Design review of the part built by this model. Coordinates are the model's own, in mm. A direction names the side the tool comes from. Coordinates: 2 decimals unless noted, no trailing zeros. Order: outer loops, then holes, each group sorted by start corner. A loop starts at its lowest first (then second) coordinate and runs counter-clockwise, first axis right, second up. Notation, with made-up numbers: M 31,63 L 58,63 A25 cw 58,78 Z; hole C 23,-19 d5. An arc over 180 degrees is marked long. Answer in a Markdown table with one row per item.
from build123d import *

# Parameters (mm, degrees)
F0_W          = 6
F0_H          = 1.5
F1_DEPTH      = 22
F2_R          = 2.5
F3_DEPTH      = 25
F3_DEPTH_BACK = 25
F4_START      = 0.5
F2_R_2        = 5
F2_R_3        = 4
F4_DEPTH      = 24.5
F2_R_4        = 1.5
F5_DEPTH      = 25
F5_DEPTH_BACK = 25
F6_DEPTH      = 25
F6_DEPTH_BACK = 1.5
F7_START      = -4
F7_DEPTH      = 21


with BuildPart() as f1:
    # F0 (on Front) → F1 (new body)
    with BuildSketch(Plane.XZ):
        with Locations((0, -4.75)):
            Rectangle(F0_W, F0_H)
        Polygon((3, -4), (10, -4), (10, 4), (-10, 4), (-10, -4), (-3, -4), align=None)
    extrude(amount=F1_DEPTH)

    # F2 (on Top) → F3 (cut, two sides)
    with BuildSketch(Plane.XY) as f3_sk:
        with Locations((0, -6.5)):
            Circle(F2_R)
    extrude(amount=F3_DEPTH, mode=Mode.SUBTRACT)
    extrude(f3_sk.sketch, amount=-F3_DEPTH_BACK, mode=Mode.SUBTRACT)

    # F2 (on Top) → F4 (cut)
    with BuildSketch(Plane.XY.offset(F4_START)):
        with Locations((0, -6.5)):
            Circle(F2_R_2)
        with Locations((0, -6.5)):
            Circle(F2_R_3, mode=Mode.SUBTRACT)
        with Locations((0, -6.5)):
            Circle(F2_R_3)
        with Locations((0, -6.5)):
            Circle(F2_R, mode=Mode.SUBTRACT)
    extrude(amount=F4_DEPTH, mode=Mode.SUBTRACT)

    # F2 (on Top) → F5 (cut, two sides)
    with BuildSketch(Plane.XY) as f5_sk:
        with Locations((-4.685, -17.2488261014)):
            Circle(F2_R_4)
        with Locations((4.685, -17.2488261014)):
            Circle(F2_R_4)
    extrude(amount=F5_DEPTH, mode=Mode.SUBTRACT)
    extrude(f5_sk.sketch, amount=-F5_DEPTH_BACK, mode=Mode.SUBTRACT)

    # F2 (on Top) → F6 (cut, two sides)
    with BuildSketch(Plane.XY) as f6_sk:
        Polygon((-1.85, -18.8856141146), (-1.85, -15.6120380883), (-4.685, -13.9752500751), (-7.52, -15.6120380883), (-7.52, -18.8856141146), (-4.685, -20.5224021277), align=None)
        with Locations((-4.685, -17.2488261014)):
            Circle(F2_R_4, mode=Mode.SUBTRACT)
        Polygon((7.52, -18.8856141146), (7.52, -15.6120380883), (4.685, -13.9752500751), (1.85, -15.6120380883), (1.85, -18.8856141146), (4.685, -20.5224021277), align=None)
        with Locations((4.685, -17.2488261014)):
            Circle(F2_R_4, mode=Mode.SUBTRACT)
    extrude(amount=-F6_DEPTH, mode=Mode.SUBTRACT)
    extrude(f6_sk.sketch, amount=F6_DEPTH_BACK, mode=Mode.SUBTRACT)

    # F2 (on Top) → F7 (cut)
    with BuildSketch(Plane.XY.offset(F7_START)):
        with Locations((0, -6.5)):
            Circle(F2_R_3)
        with Locations((0, -6.5)):
            Circle(F2_R, mode=Mode.SUBTRACT)
    extrude(amount=-F7_DEPTH, mode=Mode.SUBTRACT)


solid = f1.part
(1) Add section B-B, the plane z = -2. Give the boundary of the cut face in (x, y) (3 decimals).
Return value:
| item | result |
|---|---|
| outline | M -10,-22 L 10,-22 L 10,0 L -10,0 Z; hole M -7.52,-18.886 L -4.685,-20.522 L -1.85,-18.886 L -1.85,-15.612 L -4.685,-13.975 L -7.52,-15.612 Z; hole C 0,-6.5 d5; hole M 1.85,-18.886 L 4.685,-20.522 L 7.52,-18.886 L 7.52,-15.612 L 4.685,-13.975 L 1.85,-15.612 Z |
(2) Add section C-C, the plane y = -6.5. Give the boundary of the cut face in (x, z), and give its area (4 significant figures).
Return value:
| item | result |
|---|---|
| outline | M -10,-4 L -2.5,-4 L -2.5,0.5 L -5,0.5 L -5,4 L -10,4 Z; M 2.5,-4 L 10,-4 L 10,4 L 5,4 L 5,0.5 L 2.5,0.5 Z |
| area | 102.5 mm2 |
(3) Insertion check: pin 1 Ø6 at (x, y) = (0, -6.5) entering from +Z; pin 2 Ø4 at (x, y) = (0, -6.5) entering from +Z; pin 3 Ø2 at (x, y) = (-5, -10) entering from -Z; pin 4 Ø1.2 at (y, z) = (-2, -5) entering from +X. Each pin has a flat end and moves straight along its axis. Give the tip position at first contact, or say it passes through.
Return value:
| item | result |
|---|---|
| pin 1 | stops at z = 0.5 |
| pin 2 | passes through |
| pin 3 | stops at z = -4 |
| pin 4 | stops at x = 3 |
(4) For line 1 along X through (y, z) = (-17.75, 0); line 2 along X through (y, z) = (-6.5, 2.15); line 3 along Y through (x, z) = (2.25, -0.25), list the stretches that pass through material, from the lowest coordinate up. Write a range as from..to.
Return value:
| item | result |
|---|---|
| line 1 | x = -10..-7.52, -1.85..1.85, 7.52..10 |
| line 2 | x = -10..-5, 5..10 |
| line 3 | y = -22..-19.12, -15.38..-7.59, -5.41..0 |
(5) Add section D-D, the plane y = -13. Give the boundary of the cut face in (x, z).
Return value:
| item | result |
|---|---|
| outline | M -10,-4 L -3,-4 L -3,-5.5 L 3,-5.5 L 3,-4 L 10,-4 L 10,4 L -10,4 Z |
(6) For faces 4 (the cylindrical face through (-4, -9.5, 2.2)), 5 (the flat face through (1.85, -17, -2)), 6 (the cylindrical face through (4.36, -18.713, 2.768)), list the 3-axis set-ups (+Z, -Z, +X, -X, +Y, -Y) from which the entire face can be reached by the end or side of a thin tool; tool diameter is ignored.
Return value:
| item | result |
|---|---|
| face 4 | +Z |
| face 5 | -Z |
| face 6 | +Z, -Z |
(7) Add section A-A, the plane x = 0. Give the boundary of the cut face in (y, z), and give its area (4 significant figures).
Return value:
| item | result |
|---|---|
| outline | M -22,-5.5 L -10.5,-5.5 L -10.5,-4 L -9,-4 L -9,0.5 L -11.5,0.5 L -11.5,4 L -22,4 Z; M -4,-4 L -2.5,-4 L -2.5,-5.5 L 0,-5.5 L 0,4 L -1.5,4 L -1.5,0.5 L -4,0.5 Z |
| area | 139.5 mm2 |
(8) Draft analysis for pull direction X (two halves, no side actions). For faces 1 (the flat face through (3, -12, -5)), 2 (the flat face through (-3, -21, -5)), 3 (the flat face through (4, -19, 1.5)), state which applies: pulls with the +X half, pulls with the -X half, needs draft (parallel to the pull), parting line crosses it, or undercut.
Return value:
| item | result |
|---|---|
| face 1 | pulls with the +X half |
| face 2 | pulls with the -X half |
| face 3 | undercut |
